Verification items for the finished model (mm, model axes). A direction names the side the tool comes from. Coordinates: 2 decimals unless noted, no trailing zeros. Order: outer loops, then holes, each group sorted by start corner. A loop starts at its lowest first (then second) coordinate and runs counter-clockwise, first axis right, second up. Notation, with made-up numbers: M 25.25,59 L 45.25,59 A26 ccw 45.25,80 Z; hole C 35,76.25 d11. An arc over 180 degrees is marked long. Return JSON: item names as keys, results as strings. Group by question number.
Q1. Section check A-A, the plane z = 0. Enter the section's corners in (x, y), then the cut area to 3 significant figures.
Q2. Section check C-C, the plane x = 47.5. Enter the section's corners in (y, z), then the cut area to 3 significant figures.
Q3. Section check B-B, the plane y = 12.5. Enter the section's corners in (x, z), then the cut area to 3 significant figures.
Q4. Access from +Z, -Z, +X, -X, +Y, -Y to the whole of each face (thin tool, end or side, straight path). Record for faces 1 (the face through (30, 20, 0)), 2 (the face through (55, 5, 0)).
Q5. Thickness scan on probe 1 along Y at (x, z) = (47.5, -5); probe 2 along Z at (x, y) = (37, 8.25); probe 3 along Z at (x, y) = (36, 3.5). Record the ranges inside material, lowest first.
Q6. Go/stop test with flat-tipped pins: pin 1 Ø2.5 at (y, z) = (2, 4) entering from +X; pin 2 Ø8 at (x, z) = (53.5, 1.5) entering from -Y. Record where each tip stops, or that it passes through.
Q7. Mould release check, pull along X, two halves, no side actions. Record for faces 3 (the face through (50, 2, 0)), 4 (the face through (16.292, 9.86, 1.352)), 5 (the face through (30, 10, 9.5)): pulls with the +X half, pulls with the -X half, needs draft (parallel to the pull), parting line crosses it, or undercut.
Q8. Section check D-D, the plane z = 6.25. Enter the section's corners in (x, y), then the cut area to 3 significant figures.
from build123d import *

# Parameters (mm, degrees)
SKETCH1_W                = 60
SKETCH1_H                = 20
BOSS_EXTRUDE1_DEPTH      = 9.5
SKETCH2_W                = 10
SKETCH2_H                = 5
CUT_EXTRUDE1_DEPTH       = 20
F_9_0_9_DIAMETER_HOLE1_D = 9
M8X1_25_TAPPED_HOLE1_D   = 6.8


with BuildPart() as part:
    # Sketch1 → Boss-Extrude1 (new body, symmetric)
    with BuildSketch(Plane.XY):
        with Locations((30, 10)):
            Rectangle(SKETCH1_W, SKETCH1_H)
    extrude(amount=BOSS_EXTRUDE1_DEPTH, both=True)

    # Sketch2 → Cut-Extrude1 (cut, through all)
    with BuildSketch(Plane.XY.offset(9.5)):
        with Locations((55, 2.5)):
            Rectangle(SKETCH2_W, SKETCH2_H)
    extrude(amount=-CUT_EXTRUDE1_DEPTH, mode=Mode.SUBTRACT)

    # Ø9.0 (9) Diameter Hole1 (through all)
    with Locations(Plane(origin=(0, 20, 0), x_dir=(-1, 0, 0), z_dir=(0, 1, 0))):
        with Locations((-12, 0), (-37, 0)):
            Hole(F_9_0_9_DIAMETER_HOLE1_D / 2)

    # M8x1.25 Tapped Hole1 (through all)
    with Locations(Plane.XY.offset(9.5)):
        with Locations((47.5, 12.5)):
            Hole(M8X1_25_TAPPED_HOLE1_D / 2)


solid = part.part
Numbers:
{
 "1": {"outline": "M 0,0 L 7.5,0 L 7.5,20 L 0,20 Z; M 16.5,0 L 32.5,0 L 32.5,20 L 16.5,20 Z; M 41.5,0 L 50,0 L 50,5 L 60,5 L 60,20 L 41.5,20 Z; hole C 47.5,12.5 d6.8", "area": "754 mm2"},
 "2": {"outline": "M 0,-9.5 L 9.1,-9.5 L 9.1,9.5 L 0,9.5 Z; M 15.9,-9.5 L 20,-9.5 L 20,9.5 L 15.9,9.5 Z", "area": "251 mm2"},
 "3": {"outline": "M 0,-9.5 L 44.1,-9.5 L 44.1,9.5 L 0,9.5 Z; M 50.9,-9.5 L 60,-9.5 L 60,9.5 L 50.9,9.5 Z; hole C 12,0 d9; hole C 37,0 d9", "area": "884 mm2"},
 "4": {"face 1": "+Z, -Z, +X, -X, +Y", "face 2": "+Z, -Z, +X, -Y"},
 "5": {"probe 1": "y = 0 to 9.1, 15.9 to 20", "probe 2": "z = -9.5 to -4.5, 4.5 to 9.5", "probe 3": "z = -9.5 to -4.39, 4.39 to 9.5"},
 "6": {"pin 1": "stops at x = 50", "pin 2": "stops at y = 0"},
 "7": {"face 3": "pulls with the +X half", "face 4": "undercut", "face 5": "needs draft"},
 "8": {"outline": "M 0,0 L 50,0 L 50,5 L 60,5 L 60,20 L 0,20 Z; hole C 47.5,12.5 d6.8", "area": "1,110 mm2"}
}
